Input: part model. Units: mm. Frame: model coordinates. Face numbers are marked on the shaded views. A direction names the side the tool comes from. Coordinates: 2 decimals unless noted, no trailing zeros. Loops run counter-clockwise (first coordinate to the right, second up) from the corner with the lowest first, then second, coordinate; pieces in that order, holes last. Notation, with made-up numbers: (70.25, 33.5) - (106.25, 33.5) arc R17 ccw to (106.25, 65.5) - close; hole circle Ø7 at (11, -14). An arc over 180 degrees is marked (long way). Use one line per item in the form item = value.
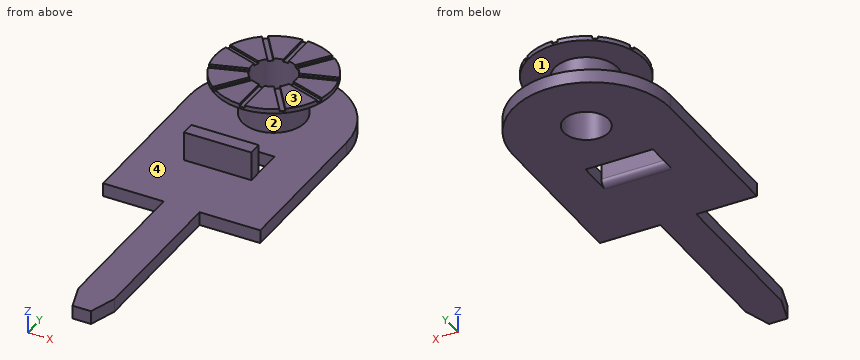
from build123d import *
from OCP.BRepFilletAPI import BRepFilletAPI_MakeChamfer

# Parameters (mm, degrees)
SKETCH1_R           = 0.5
SKETCH1_W           = 1.5
SKETCH1_H           = 0.8
BOSS_EXTRUDE1_DEPTH = 0.15
FILLET1_RADIUS      = 1.75
FILLET1_LENGTH      = 0.3
CHAMFER1_SIZE       = 0.6
CHAMFER1_SIZE2      = 0.194951818
SKETCH2_W           = 1.5
SKETCH2_H           = 0.3
BOSS_EXTRUDE2_DEPTH = 0.8
BOSS_EXTRUDE3_START = -1
BOSS_EXTRUDE3_DEPTH = 1.5
SKETCH4_R           = 0.7
SKETCH4_R_2         = 0.5
BOSS_EXTRUDE4_DEPTH = 1
BOSS_EXTRUDE5_START = 1
SKETCH5_R           = 1.3
SKETCH5_R_2         = 0.5
BOSS_EXTRUDE5_DEPTH = 0.1
CUT_EXTRUDE1_START  = 1.1
CUT_EXTRUDE1_DEPTH  = 0.05


with BuildPart() as part:
    # Sketch1 → Boss-Extrude1 (new, symmetric)
    with BuildSketch(Plane.XY):
        Polygon((-2.15, -5.3), (-3.5, -5.3), (-3.5, 0), (0, 0), (0, -5.3), (-1.35, -5.3), (-1.35, -9.4), (-2.15, -9.4), align=None)
        with Locations((-1.75, -1.52)):
            Circle(SKETCH1_R, mode=Mode.SUBTRACT)
        with Locations((-1.75, -3.27)):
            Rectangle(SKETCH1_W, SKETCH1_H, mode=Mode.SUBTRACT)
    extrude(amount=BOSS_EXTRUDE1_DEPTH, both=True)

    # Fillet1: full round fillet: the end face becomes a half cylinder, R = half its width
    fillet1_face = Plane((-1.75, 0, 0), x_dir=(0, 0, 1), z_dir=(0, 1, 0))  # on the end face: x along it, z out of the body
    fillet1_slab = fillet1_face.offset(-FILLET1_RADIUS / 2) * Box(FILLET1_LENGTH, 2 * FILLET1_RADIUS, FILLET1_RADIUS, mode=Mode.PRIVATE)  # the body's end, R deep
    fillet1_round = Plane((-1.75, -1.75, 0), x_dir=(0, 1, 0), z_dir=(0, 0, 1)) * Cylinder(FILLET1_RADIUS, FILLET1_LENGTH, mode=Mode.PRIVATE)  # its axis R under the face
    add(fillet1_slab - fillet1_round, mode=Mode.SUBTRACT)

    # Chamfer1: one chamfer whose edges measure the first distance from different faces: ONE call of the kernel's chamfer builder (chamfer() names one face for all edges)
    chamfer1_edges_1 = [part.edges().sort_by_distance(p)[0] for p in [
        (-1.35, -9.4, 0),
    ]]
    chamfer1_side_1 = [part.faces().sort_by_distance(p)[0] for p in [
        (-1.35, -7.35, 0),
    ]]
    chamfer1_edges_2 = [part.edges().sort_by_distance(p)[0] for p in [
        (-2.15, -9.4, 0),
    ]]
    chamfer1_side_2 = [part.faces().sort_by_distance(p)[0] for p in [
        (-2.15, -7.35, 0),
    ]]
    chamfer1 = BRepFilletAPI_MakeChamfer(part.part.solid().wrapped)
    for e in chamfer1_edges_1:
        chamfer1.Add(CHAMFER1_SIZE, CHAMFER1_SIZE2, e.wrapped, chamfer1_side_1[0].wrapped)  # the first distance lies on this face
    for e in chamfer1_edges_2:
        chamfer1.Add(CHAMFER1_SIZE, CHAMFER1_SIZE2, e.wrapped, chamfer1_side_2[0].wrapped)  # the first distance lies on this face
    add(Compound.cast(chamfer1.Shape()), mode=Mode.REPLACE)

    # Sketch2 → Boss-Extrude2 (add)
    with BuildSketch(Plane.XY):
        with Locations((-1.75, -3.67)):
            Rectangle(SKETCH2_W, SKETCH2_H)
    extrude(amount=BOSS_EXTRUDE2_DEPTH)

    # Sketch3 → Boss-Extrude3 (add)
    with BuildSketch(Plane(origin=(0, 0, 0), x_dir=(0, 0, -1), z_dir=(1, 0, 0)).offset(BOSS_EXTRUDE3_START)):
        with BuildLine():
            Line((0.15, -3.67), (0, -3.67))
            Line((0, -3.67), (0, -3.52))
            ThreePointArc((0, -3.52), (0.106066017, -3.563933983), (0.15, -3.67))
        make_face()
    extrude(amount=-BOSS_EXTRUDE3_DEPTH)

    # Sketch4 → Boss-Extrude4 (add)
    with BuildSketch(Plane.XY):
        with Locations(Location((-1.75, -1.52, 0), (0, 0, 180))):
            Circle(SKETCH4_R)
        with Locations((-1.75, -1.52)):
            Circle(SKETCH4_R_2, mode=Mode.SUBTRACT)
    extrude(amount=BOSS_EXTRUDE4_DEPTH)

    # Sketch5 → Boss-Extrude5 (add)
    with BuildSketch(Plane.XY.offset(BOSS_EXTRUDE5_START)):
        with Locations((-1.75, -1.52)):
            Circle(SKETCH5_R)
        with Locations((-1.75, -1.52)):
            Circle(SKETCH5_R_2, mode=Mode.SUBTRACT)
    extrude(amount=BOSS_EXTRUDE5_DEPTH)

    # Sketch6 → Cut-Extrude1 (cut)
    with BuildSketch(Plane.XY.offset(CUT_EXTRUDE1_START)):
        Polygon((-1.75, -1.417921903), (-1.69, -1.335338988), (-1.69, -0.22), (-1.81, -0.22), (-1.81, -1.335338988), align=None)
        Polygon((-1.81, -1.437417085), (-1.81, -1.335338988), (-2.465579808, -0.433010792), (-2.562661848, -0.503545022), (-1.907082039, -1.405873218), align=None)
        Polygon((-1.944164079, -1.52), (-1.847082039, -1.488456133), (-1.907082039, -1.405873218), (-2.967832452, -1.061214516), (-3.004914491, -1.175341298), align=None)
        Polygon((-2.967832452, -1.978785484), (-1.907082039, -1.634126782), (-1.847082039, -1.551543867), (-1.944164079, -1.52), (-3.004914491, -1.864658702), align=None)
        Polygon((-1.69, -1.437417085), (-1.592917961, -1.405873218), (-0.937338152, -0.503545022), (-1.034420192, -0.433010792), (-1.69, -1.335338988), align=None)
        Polygon((-1.555835921, -1.52), (-0.495085509, -1.175341298), (-0.532167548, -1.061214516), (-1.592917961, -1.405873218), (-1.652917961, -1.488456133), align=None)
        Polygon((-0.495085509, -1.864658702), (-1.555835921, -1.52), (-1.652917961, -1.551543867), (-1.592917961, -1.634126782), (-0.532167548, -1.978785484), align=None)
        Polygon((-1.81, -1.704661012), (-1.81, -1.602582915), (-1.907082039, -1.634126782), (-2.562661848, -2.536454978), (-2.465579808, -2.606989208), align=None)
        Polygon((-0.937338152, -2.536454978), (-1.592917961, -1.634126782), (-1.69, -1.602582915), (-1.69, -1.704661012), (-1.034420192, -2.606989208), align=None)
        Polygon((-1.69, -2.82), (-1.69, -1.704661012), (-1.75, -1.622078097), (-1.81, -1.704661012), (-1.81, -2.82), align=None)
    extrude(amount=-CUT_EXTRUDE1_DEPTH, mode=Mode.SUBTRACT)


solid = part.part
Q1. Cut plane A-A, the plane y = -3.25. Return loops of the section in (x, z).
Check values:
outline = (-3.5, -0.15) - (-2.5, -0.15) - (-2.5, 0.15) - (-3.5, 0.15) - close; (-1, -0.15) - (0, -0.15) - (0, 0.15) - (-1, 0.15) - close
Q2. Pull-direction query (Y, two-part tool) for the marked faces 1 and 2; classes: pulls with the +Y half, pulls with the -Y half, needs draft (parallel to the pull), parting line crosses it, or undercut.
Check values:
face_1 = needs draft
face_2 = undercut
Q3. Cut plane D-D, the plane y = -1.52. Return loops of the section in (x, z).
Check values:
outline = (-3.48, -0.15) - (-2.25, -0.15) - (-2.25, 1.1) - (-3.05, 1.1) - (-3.05, 1) - (-2.45, 1) - (-2.45, 0.15) - (-3.48, 0.15) - close; (-1.25, -0.15) - (-0.02, -0.15) - (-0.02, 0.15) - (-1.05, 0.15) - (-1.05, 1) - (-0.45, 1) - (-0.45, 1.1) - (-1.25, 1.1) - close
Q4. Cut plane B-B, the plane z = 0.25. Return loops of the section in (x, y), then the cut area to 3 significant figures.
Check values:
outline = (-2.5, -3.82) - (-1, -3.82) - (-1, -3.52) - (-2.5, -3.52) - close; circle Ø1.4 at (-1.75, -1.52); hole circle Ø1 at (-1.75, -1.52)
area = 1.20 mm²
Q5. Cut plane C-C, the plane x = -0.35. Return loops of the section in (y, z), then the cut area to 3 significant figures.
Check values:
outline = (-5.3, -0.15) - (-0.7, -0.15) - (-0.7, 0.15) - (-5.3, 0.15) - close
area = 1.38 mm²
Q6. First-contact query: P1, Ø0.6, axis at x = -2, z = 0, coming from the +Y side. Flat tip, straight axial feed; report the tip coordinate or a pass-through.
Check values:
P1 = 0
Q7. Ray query, line 1 along Y through (x, z) = (-1.75, 0.6); line 2 along Y through (x, z) = (-2.15, 0.4); line 3 along X through (y, z) = (-1.52, 0.5). Return the intervals inside material, ascending. Write a range as [from, to].
Check values:
line_1 = [-3.82, -3.52], [-2.22, -2.02], [-1.02, -0.82]
line_2 = [-3.82, -3.52], [-2.09, -1.82], [-1.22, -0.95]
line_3 = [-2.45, -2.25], [-1.25, -1.05]
Q8. Set-up query: the marked faces 3 and 4. Return all of +Z, -Z, +X, -X, +Y, -Y with unobstructed straight access to the full face (end or side cutting, diameter ignored); none if empty.
Check values:
face_3 = +Z, +X, -X, +Y, -Y
face_4 = none
